Geometry check sheet. Reference: the model listing, model coordinates, mm. A direction names the side the tool comes from. Round coordinates to 2 decimals unless told otherwise and drop trailing zeros. Write each loop counter-clockwise with the first axis right and the second up, starting at its lowest first coordinate (ties: lowest second). Pieces come first, ordered by that corner, then holes. Notation, with made-up numbers: (59.25, -3) -> (76.25, -3) arc R22 ccw to (76.25, 28) -> close; hole circle Ø2 at (-36.5, 24.25). An arc over 180 degrees is marked (long way). Put each result on its own line as item: value. Start each with the question number.
Autodesk Inventor part; units mm, degrees
ref_plane "YZ Plane" through (0, 0, 0) normal (1, 0, 0) x (0, 1, 0)
ref_plane "XZ Plane" through (0, 0, 0) normal (0, 1, 0) x (-1, 0, 0)
ref_plane "XY Plane" through (0, 0, 0) normal (0, 0, 1) x (1, 0, 0)
sketch "スケッチ1" plane through (0, 0, 0) normal (0, 0, 1) x (1, 0, 0)
  circle A0 centre (0, 0) radius 2
  dimension "d0" = 4
extrude "押し出し1" add sketch "スケッチ1" along normal blind 8
sketch "スケッチ2" plane through (0, 0, 8) normal (0, 0, 1) x (1, 0, 0)
  circle A0 centre (0, 0) radius 2
  circle A1 centre (0, 0) radius 3
  dimension "d3" = 6
extrude "押し出し2" add sketch "スケッチ2" along normal blind 2 contours A0 | A1
fillet "フィレット1" radius 2 1 edges at (-3, 0, 10)
properties part number "M4ボタンボルト8" material "鋼、高強度、低合金"
(1) Sectioned sample at A-A (z = 2). Record the cut outline in (x, y).
(2) Go/stop test with flat-tipped pins: pin 1 Ø3 at (y, z) = (-2, 7) entering from -X; pin 2 Ø1.5 at (y, z) = (2, 4) entering from +X; pin 3 Ø1 at (x, y) = (-2, -2.5) entering from +Z. Record where each tip stops, or that it passes through.
(3) Material ranges on L1, parallel to Y at x = 0, z = 7.5; L2, parallel to Y at x = 0.75, z = 0.75; L3, parallel to Z at x = 1.25, y = 2, recorded low to high. Write a range as from..to.
(4) Set-up check for faces 1 (the flat face through (0, 0, 10)), 2 (the cylindrical face through (0, 2, 4)): record each of +Z, -Z, +X, -X, +Y, -Y from which the full face is reachable in a straight line by a thin tool's end or side.
Found:
1. outline: circle Ø4 at (0, 0)
2. pin 1: x = -2.87
2. pin 2: x = 1.56
2. pin 3: z = 9.05
3. L1: -2..2
3. L2: -1.85..1.85
3. L3: 8..9.47
4. face 1: +Z, +X, -X, +Y, -Y
4. face 2: -Z
